Autodesk Inventor part; units mm, degrees
ref_plane "YZ Plane" through (0, 0, 0) normal (1, 0, 0) x (0, 1, 0)
ref_plane "XZ Plane" through (0, 0, 0) normal (0, 1, 0) x (-1, 0, 0)
ref_plane "XY Plane" through (0, 0, 0) normal (0, 0, 1) x (1, 0, 0)
sketch "Sketch1" plane through (0, 0, 0) normal (0, 1, 0) x (-1, 0, 0)
  line L0 (0, 0) -> (0, -53)
  circle A0 centre (0, 0) radius 4
  circle A1 centre (0, -53) radius 4
  line L1 (0, 8.5) -> (10, 8.5)
  line L2 (10, 8.5) -> (-10, 8.5)
  line L3 (-10, 8.5) -> (-10, -61.5)
  line L4 (-10, -61.5) -> (10, -61.5)
  line L5 (10, -61.5) -> (10, 8.5)
  dimension "d0" = 53
  dimension "d1" = 8
  dimension "d2" = 8
  dimension "d3" = 8.5
  dimension "d4" = 10
  dimension "d8" = 10
  dimension "d9" = 10
  dimension "d10" = 70
extrude "Extrusion1" add sketch "Sketch1" along normal blind 21
fillet "Fillet1" radius 2 4 edges at (10, 10.5, 8.5) (-10, 10.5, 8.5) (10, 10.5, -61.5) (-10, 10.5, -61.5)
properties part number "Bearing Seats 10mm (Short)"
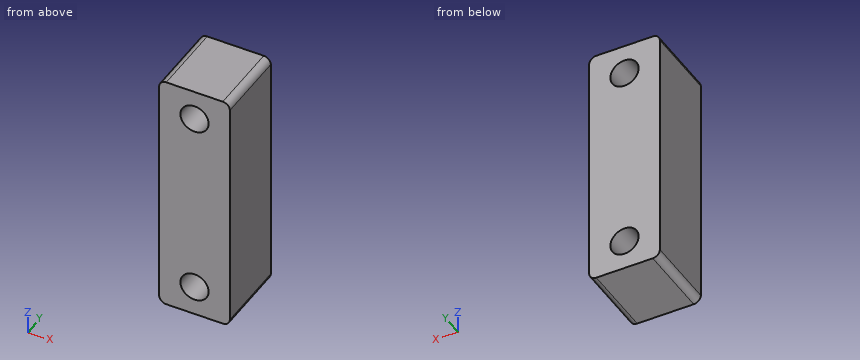
Could you check a few things on this model? Use its own coordinates, in mm. Give positions to 0.01 mm unless a question says otherwise; leave off trailing zeros. Order: outer loops, then holes, each group sorted by start corner. A loop starts at its lowest first (then second) coordinate and runs counter-clockwise, first axis right, second up. Notation, with made-up numbers: (69.5, -13.5) - (118.5, -13.5) arc R20 cw to (118.5, 10.5) - close; hole circle Ø7 at (37.5, 19). An arc over 180 degrees is marked (long way). One line per item, written item: value. Start each with the question number.
1. Imagine slicing it at A-A on z = -53. List the corners of the cut face in (x, y) for me, plus the area to 3 significant figures.
2. If I drill on probe 1 along Z at (x, y) = (0, 15.25); probe 2 along Z at (x, y) = (-3, 15); probe 3 along X at (y, z) = (12.5, 0), over which ranges is the centre line in solid material (lowest first)?
3. Imagine slicing it at B-B on x = 0. List the corners of the cut face in (y, z) for me.
4. Imagine slicing it at C-C on y = 10.5. List the corners of the cut face in (x, z) for me.
5. Imagine slicing it at D-D on x = -3.25. List the corners of the cut face in (y, z) for me.
Values:
1. outline: (-10, 0) - (-4, 0) - (-4, 21) - (-10, 21) - close; (4, 0) - (10, 0) - (10, 21) - (4, 21) - close
1. area: 252 mm²
2. probe 1: -61.5 to -57, -49 to -4, 4 to 8.5
2. probe 2: -61.5 to -55.65, -50.35 to -2.65, 2.65 to 8.5
2. probe 3: -10 to -4, 4 to 10
3. outline: (0, -61.5) - (21, -61.5) - (21, -57) - (0, -57) - close; (0, -49) - (21, -49) - (21, -4) - (0, -4) - close; (0, 4) - (21, 4) - (21, 8.5) - (0, 8.5) - close
4. outline: (-10, -59.5) arc R2 ccw to (-8, -61.5) - (8, -61.5) arc R2 ccw to (10, -59.5) - (10, 6.5) arc R2 ccw to (8, 8.5) - (-8, 8.5) arc R2 ccw to (-10, 6.5) - close; hole circle Ø8 at (0, -53); hole circle Ø8 at (0, 0)
5. outline: (0, -61.5) - (21, -61.5) - (21, -55.33) - (0, -55.33) - close; (0, -50.67) - (21, -50.67) - (21, -2.33) - (0, -2.33) - close; (0, 2.33) - (21, 2.33) - (21, 8.5) - (0, 8.5) - close
